from build123d import *

# Parameters (mm, degrees)
F1_DEPTH        = 9.525
F2_R            = 25.4
F3_DEPTH        = 12.7
F4_W            = 12.7
F4_H            = 12.7
F5_DEPTH        = 12.7
F6_R            = 3.701609
F7_DEPTH        = 6.35
F9_D            = 6.35
F11_D           = 6.35
F11_CBORE_D     = 10.16
F11_CBORE_DEPTH = 3.175


with BuildPart() as f1:
    # F0 (on Front) → F1 (new body, symmetric)
    with BuildSketch(Plane.XZ):
        with BuildLine():
            Line((-72.97454, 0), (-44.45, 0))
            ThreePointArc((-44.45, 0), (31.430896, -31.430896), (0, 44.45))
            Line((0, 44.45), (0, 72.97454))
            Line((0, 72.97454), (-72.97454, 0))
        make_face()
    extrude(amount=F1_DEPTH, both=True)

    # F2 (on face) → F3 (join)
    with BuildSketch(Plane.XZ.offset(9.525)):
        Circle(F2_R)
    extrude(amount=F3_DEPTH)

    # F4 (on face) → F5 (join)
    with BuildSketch(Plane.XZ.offset(22.225)):
        Rectangle(F4_W, F4_H)
    extrude(amount=F5_DEPTH)

    # F6 (on face) → F7 (join)
    with BuildSketch(Plane.XZ.offset(34.925)):
        Circle(F6_R)
    extrude(amount=F7_DEPTH)

    # F9 (through all)
    with Locations(Plane.XZ.offset(41.275)):
        with Locations((0, 0)):
            Hole(F9_D / 2)

    # F11 (through all)
    with Locations(Plane.XZ.offset(22.225)):
        with Locations((-15.339203, 0)):
            CounterBoreHole(F11_D / 2, F11_CBORE_D / 2, F11_CBORE_DEPTH)


solid = f1.part
The model under review builds one solid part; all positions refer to its coordinate system, in mm. A direction names the side the tool comes from. Round coordinates to 2 decimals unless told otherwise and drop trailing zeros. Write each loop counter-clockwise with the first axis right and the second up, starting at its lowest first coordinate (ties: lowest second). Pieces come first, ordered by that corner, then holes. Notation, with made-up numbers: (42, 41) -> (54, 41) arc R16 cw to (54, 65) -> close; hole circle Ø4 at (-34.75, 12.25). An arc over 180 degrees is marked (long way). Answer as a JSON object with one key per item and string values.
1. The part is to be moulded in two halves that separate along Z. For faces 6 (the face through (0, -28, -6.35)), 7 (the face through (3, -34.925, -3)), 8 (the face through (-18.27, -4.56, -1.22)), say which applies: pulls with the +Z half, pulls with the -Z half, needs draft (parallel to the pull), parting line crosses it, or undercut.
Results found:
{"face 6": "pulls with the -Z half", "face 7": "needs draft", "face 8": "undercut"}
2. Machinability: for faces 1 (the face through (-6.35, -28, 0)), 2 (the face through (-28, -9.525, 2)), 3 (the face through (-59, 0, 0)), 4 (the face through (6.35, -28, 0)), 5 (the face through (0, -28, 6.35)), which of the approach directions +Z, -Z, +X, -X, +Y, -Y give a long, thin tool a straight path to every point of the face, cutting with its end or side? Answer none if there is none.
Results found:
{"face 1": "+Z, -Z, -X, -Y", "face 2": "-Y", "face 3": "-Z, -X, +Y, -Y", "face 4": "+Z, -Z, +X, -Y", "face 5": "+Z, +X, -X, -Y"}
3. We need section D-D on x = 30.5. State the section outline as (y, z) points (3 decimals).
Results found:
{"outline": "(-9.525, -32.335) -> (9.525, -32.335) -> (9.525, 32.335) -> (-9.525, 32.335) -> close"}
4. Clearance check with flat-ended pins moving along their axes: pin 1 (6.5 mm diameter, centred on y = -31, z = -0.5, fed in from -X); pin 2 (3 mm diameter, centred on x = 31, z = -30.5, fed in from -Y) (3 decimals); pin 3 (6.5 mm diameter, centred on x = -0.5, z = -0.5, fed in from -Y) (3 decimals); pin 4 (9.5 mm diameter, centred on y = 0, z = 52.5, fed in from +X). State where each tip first meets the part, or that it passes through.
Results found:
{"pin 1": "stops at x = -6.35", "pin 2": "stops at y = -9.525", "pin 3": "stops at y = -41.275", "pin 4": "stops at x = 0"}
5. To check wall thickness, follow line 1 along Z through (x, y) = (0, -18) (3 decimals); line 2 along Z through (x, y) = (4, -24.5); line 3 along Z through (x, y) = (-15.5, 7.5). State the ranges of each line that lie inside material, in increasing order.
Results found:
{"line 1": "z = -25.4 to -3.175, 3.175 to 25.4", "line 2": "z = -6.35 to 6.35", "line 3": "z = -41.66 to -3.17, 3.17 to 57.47"}
6. We need section A-A on y = -11. State the section outline as (x, z) points (3 decimals).
Results found:
{"outline": "circle Ø50.8 at (0, 0); hole circle Ø6.35 at (-15.339, 0); hole circle Ø6.35 at (0, 0)"}
7. We need section B-B on z = 17.5. State the section outline as (x, y) points (1 decimal).
Results found:
{"outline": "(-55.5, -9.5) -> (-18.4, -9.5) -> (-18.4, -22.2) -> (18.4, -22.2) -> (18.4, -9.5) -> (40.9, -9.5) -> (40.9, 9.5) -> (-55.5, 9.5) -> close"}
8. We need section C-C on y = 6. State the section outline as (x, z) points (3 decimals).
Results found:
{"outline": "(-72.975, 0) -> (-44.45, 0) arc R44.45 ccw (long way) to (0, 44.45) -> (0, 72.975) -> close; hole circle Ø6.35 at (-15.339, 0); hole circle Ø6.35 at (0, 0)"}
